Source: three-view drawing plus pictorial views. Frame: mm from the lowest corner of the part. A direction names the side the tool comes from. Give positions to 0.01 mm unless a question says otherwise; leave off trailing zeros. Loops run counter-clockwise (first coordinate to the right, second up) from the corner with the lowest first, then second, coordinate; pieces in that order, holes last.
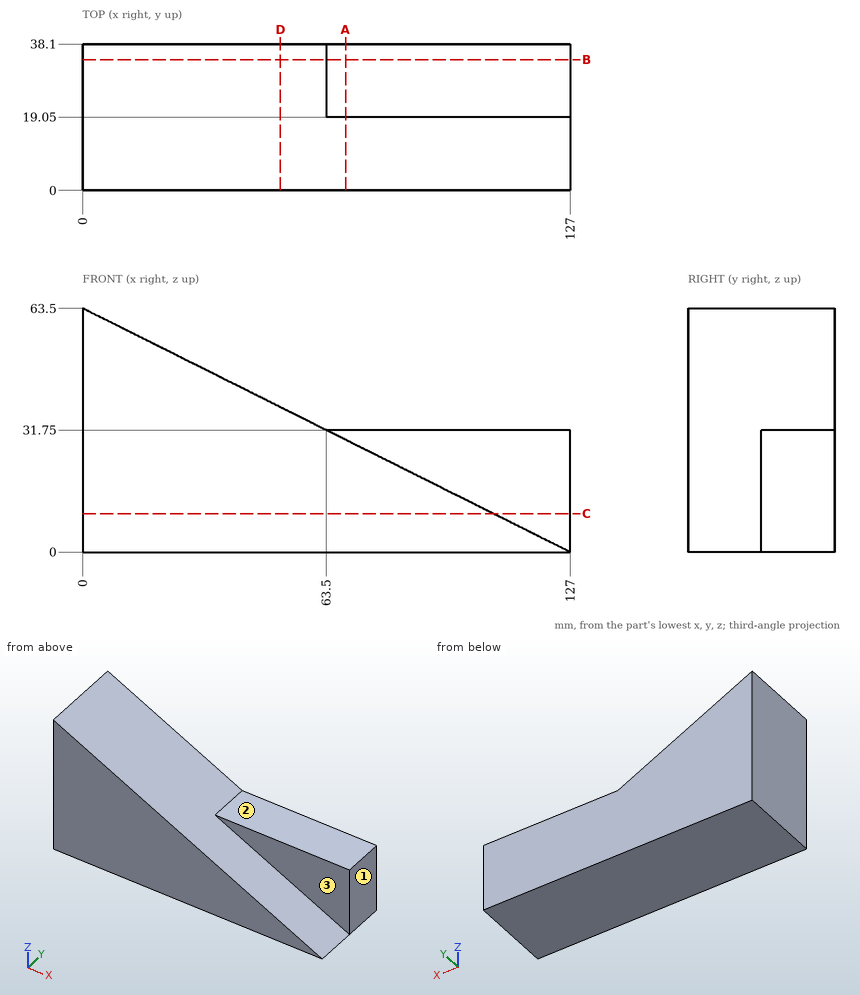
(1) Cut plane B-B (y = 34). Return the cut outline in (x, z).
Values follow:
outline: (0, 0) - (127, 0) - (127, 31.75) - (63.5, 31.75) - (0, 63.5) - close
(2) Cut plane C-C (z = 10). Return the cut outline in (x, y), and give its area (3 significant figures).
Values follow:
outline: (0, 0) - (107, 0) - (107, 19.05) - (127, 19.05) - (127, 38.1) - (0, 38.1) - close
area: 4,460 mm2
(3) Pin query (flat end, axial travel): pin 1 Ø9.5 at (x, y) = (102.5, 27.5) entering from +Z; pin 2 Ø10 at (y, z) = (4, 51) entering from +X. Return the tip coordinate at first contact, or that it passes through.
Values follow:
pin 1: stops at z = 31.75
pin 2: stops at x = 35
(4) Cut plane A-A (x = 68.5). Return the cut outline in (y, z), and give its area (3 significant figures).
Values follow:
outline: (0, 0) - (38.1, 0) - (38.1, 31.75) - (19.05, 31.75) - (19.05, 29.25) - (0, 29.25) - close
area: 1,160 mm2
(5) Cut plane D-D (x = 51.5). Return the cut outline in (y, z), and give its area (3 significant figures).
Values follow:
outline: (0, 0) - (38.1, 0) - (38.1, 37.75) - (0, 37.75) - close
area: 1,440 mm2
(6) Reachability of the marked faces 1, 2 and 3 from +Z, -Z, +X, -X, +Y, -Y: full face, straight path, thin tool, end or side. Return the list, or none.
Values follow:
face 1: +Z, -Z, +X, +Y, -Y
face 2: +Z, +X, +Y, -Y
face 3: +Z, +X, -Y
(7) Ray query, probe 1 along Z at (x, y) = (98.5, 19.5); probe 2 along Y at (x, z) = (98, 24); probe 3 along Z at (x, y) = (77, 10). Return the intervals inside material, ascending.
Values follow:
probe 1: z = 0 to 31.75
probe 2: y = 19.05 to 38.1
probe 3: z = 0 to 25
